```python
from build123d import *

# Parameters (mm, degrees)
SKETCH_1_W          = 90
SKETCH_1_H          = 14
EXTRUDE_1_DEPTH     = 1
EXTRUDE_2_DEPTH     = 1
SKETCH_4_W          = 40
SKETCH_4_H          = 14
SKETCH_4_W_2        = 19
EXTRUDE_3_DEPTH     = 1
SKETCH_7_R          = 1.6
CUT_EXTRUDE_1_DEPTH = 10
SKETCH_9_R          = 1.6
CUT_EXTRUDE_3_DEPTH = 10
EXTRUDE_4_DEPTH     = 1
CUT_EXTRUDE_4_DEPTH = 10
SKETCH_13_R         = 1.6
CUT_EXTRUDE_5_DEPTH = 10
CUT_EXTRUDE_6_DEPTH = 10
FILLET_1_R          = 5
FILLET_2_R          = 1
SKETCH_15_W         = 16
SKETCH_15_H         = 16
CUT_EXTRUDE_7_DEPTH = 10
FILLET_3_R          = 1


with BuildPart() as part:
    # 草图1 → 凸台-拉伸1 (new body)
    with BuildSketch(Plane.XY):
        with Locations((0, -3)):
            Rectangle(SKETCH_1_W, SKETCH_1_H)
    extrude(amount=EXTRUDE_1_DEPTH)

    # 草图2 → 凸台-拉伸2 (add)
    with BuildSketch(Plane.XY.offset(1)):
        Polygon((-85, 8.2), (-85, 4), (64, 4), (64, 118), (-114, 98), (-114, 8.2), align=None)
    extrude(amount=-EXTRUDE_2_DEPTH)

    # 草图4 → 凸台-拉伸3 (add)
    with BuildSketch(Plane.XY.offset(1)):
        with Locations((-65, -3)):
            Rectangle(SKETCH_4_W, SKETCH_4_H)
        with Locations((54.5, -3)):
            Rectangle(SKETCH_4_W_2, SKETCH_4_H)
    extrude(amount=-EXTRUDE_3_DEPTH)

    # 草图7 → 切除-拉伸1 (cut)
    with BuildSketch(Plane.XY.offset(1)):
        with Locations((45, 0)):
            Circle(SKETCH_7_R)
        with Locations((25, 0)):
            Circle(SKETCH_7_R)
        with Locations((-66, 0)):
            Circle(SKETCH_7_R)
        with Locations((-46, 0)):
            Circle(SKETCH_7_R)
    extrude(amount=-CUT_EXTRUDE_1_DEPTH, mode=Mode.SUBTRACT)

    # 草图9 → 切除-拉伸3 (cut)
    with BuildSketch(Plane(origin=(0, 0, 0), x_dir=(-1, 0, 0), z_dir=(0, 0, -1))):
        with Locations((110, 58.1)):
            Circle(SKETCH_9_R)
        with Locations((110, 38.1)):
            Circle(SKETCH_9_R)
    extrude(amount=-CUT_EXTRUDE_3_DEPTH, mode=Mode.SUBTRACT)

    # 草图10 → 凸台-拉伸4 (add)
    with BuildSketch(Plane.XY.offset(1)):
        Polygon((-114, 98), (-114, 118), (64, 118), align=None)
    extrude(amount=-EXTRUDE_4_DEPTH)

    # 草图11 → 切除-拉伸4 (cut)
    with BuildSketch(Plane.XY.offset(1)):
        Polygon((-44, 118), (-114, 118), (-114, 99), align=None)
    extrude(amount=-CUT_EXTRUDE_4_DEPTH, mode=Mode.SUBTRACT)

    # 草图13 → 切除-拉伸5 (cut)
    with BuildSketch(Plane.XY.offset(1)):
        with Locations((-1, 115)):
            Circle(SKETCH_13_R)
        with Locations((19, 115)):
            Circle(SKETCH_13_R)
        with Locations((-75.396749016, 106.369478786)):
            Circle(SKETCH_13_R)
        with Locations((-94.698374508, 101.130466152)):
            Circle(SKETCH_13_R)
    extrude(amount=-CUT_EXTRUDE_5_DEPTH, mode=Mode.SUBTRACT)

    # 草图14 → 切除-拉伸6 (cut)
    with BuildSketch(Plane(origin=(0, 0, 0), x_dir=(-1, 0, 0), z_dir=(0, 0, -1))):
        with BuildLine():
            Line((-94, 97), (-34, 97))
            ThreePointArc((-34, 97), (-14, 77), (-34, 57))
            Line((-34, 57), (-94, 57))
            ThreePointArc((-94, 57), (-114, 77), (-94, 97))
        make_face()
    extrude(amount=-CUT_EXTRUDE_6_DEPTH, mode=Mode.SUBTRACT)

    # 圆角1
    fillet_1_edges = [part.edges().sort_by_distance(p)[0] for p in [
        (64, 57, 0.5),
        (64, 97, 0.5),
    ]]
    fillet(fillet_1_edges, radius=FILLET_1_R)

    # 圆角2
    fillet_2_edges = [part.edges().sort_by_distance(p)[0] for p in [
        (-44, 118, 0.5),
        (-114, 99, 0.5),
        (-114, 8.2, 0.5),
        (64, 118, 0.5),
        (-85, 8.2, 0.5),
        (-85, -10, 0.5),
        (64, -10, 0.5),
    ]]
    fillet(fillet_2_edges, radius=FILLET_2_R)

    # 草图15 → 切除-拉伸7 (cut)
    with BuildSketch(Plane.XY.offset(1)):
        with Locations((-10.5, 12)):
            Rectangle(SKETCH_15_W, SKETCH_15_H)
    extrude(amount=-CUT_EXTRUDE_7_DEPTH, mode=Mode.SUBTRACT)

    # 圆角3
    fillet_3_edges = [part.edges().sort_by_distance(p)[0] for p in [
        (-2.5, 20, 0.5),
        (-2.5, 4, 0.5),
        (-18.5, 4, 0.5),
        (-18.5, 20, 0.5),
    ]]
    fillet(fillet_3_edges, radius=FILLET_3_R)


solid = part.part
```
Check sheet for the modelled part. Datum: model origin and axes. Units: mm. A direction names the side the tool comes from. Coordinates: 2 decimals unless noted, no trailing zeros. Write each loop counter-clockwise with the first axis right and the second up, starting at its lowest first coordinate (ties: lowest second). Pieces come first, ordered by that corner, then holes. Notation, with made-up numbers: (81, 21.5) - (115, 21.5) arc R6 cw to (115, 32.5) - close; hole circle Ø1 at (-18, 7). An arc over 180 degrees is marked (long way). One line per question, with ' | ' between items.
Item 1: Mould release check, pull along Y, two halves, no side actions. Record for faces 1 (the face through (-79.18, 108.45, 0.51)), 2 (the face through (14.005, 77.44, 0.493)), 3 (the face through (-24, 55, 0)): pulls with the +Y half, pulls with the -Y half, needs draft (parallel to the pull), parting line crosses it, or undercut.
Determined:
face 1: pulls with the +Y half | face 2: undercut | face 3: needs draft
Item 2: Sectioned sample at A-A on z = 0.25. Give the number of separate pieces and of enclosed holes in the cut face, plus the area to 3 significant figures.
Determined:
separate pieces: 1 | enclosed holes: 11 | area: 19,400 mm2
Item 3: Sectioned sample at B-B on y = 77. Record the boundary of the cut face in (x, z), plus the area to 3 significant figures.
Determined:
outline: (-114, 0) - (14, 0) - (14, 1) - (-114, 1) - close | area: 128 mm2
Item 4: Access from +Z, -Z, +X, -X, +Y, -Y to the whole of each face (thin tool, end or side, straight path). Record for faces 4 (the face through (62.57, 55.5, 0.51)), 5 (the face through (-24, 55, 1)).
Determined:
face 4: +Z, -Z, +X | face 5: +Z, +X, -X, +Y, -Y
Item 5: Thickness scan on line 1 (Y direction, x = 45, z = 0.75); line 2 (Y direction, x = -10, z = 0.2); line 3 (Y direction, x = 44.5, z = 0.8). Record the ranges inside material, lowest first. Write a range as [from, to].
Determined:
line 1: y = [-10, -1.6], [1.6, 57], [97, 118] | line 2: y = [-10, 4], [20, 118] | line 3: y = [-10, -1.52], [1.52, 57], [97, 118]
Item 6: Sectioned sample at C-C on x = -91. Record the boundary of the cut face in (y, z), plus the area to 3 significant figures.
Determined:
outline: (8.2, 0) - (105.24, 0) - (105.24, 1) - (8.2, 1) - close | area: 97.0 mm2
